Autodesk Inventor part; units mm, degrees
ref_plane "YZ Plane" through (0, 0, 0) normal (1, 0, 0) x (0, 1, 0)
ref_plane "XZ Plane" through (0, 0, 0) normal (0, 1, 0) x (-1, 0, 0)
ref_plane "XY Plane" through (0, 0, 0) normal (0, 0, 1) x (1, 0, 0)
sketch "Sketch1" plane through (0, 0, 0) normal (0, 1, 0) x (-1, 0, 0)
  circle A0 centre (0, 0) radius 95.25 construction
  circle A1 centre (0, 0) radius 120.65 construction
  line L0 (-69.6573, -120.65) -> (-139.3146, 0)
  line L1 (-139.3146, 0) -> (-69.6573, 120.65)
  line L2 (-69.6573, 120.65) -> (69.6573, 120.65)
  line L3 (69.6573, 120.65) -> (139.3146, 0)
  line L4 (139.3146, 0) -> (69.6573, -120.65)
  line L5 (69.6573, -120.65) -> (-69.6573, -120.65)
  line L6 (142.4896, 0) -> (71.2448, 123.3996)
  line L7 (71.2448, 123.3996) -> (-71.2448, 123.3996)
  line L8 (-71.2448, 123.3996) -> (-142.4896, 0)
  line L9 (-142.4896, 0) -> (-71.2448, -123.3996)
  line L10 (-71.2448, -123.3996) -> (71.2448, -123.3996)
  line L11 (71.2448, -123.3996) -> (142.4896, 0)
  dimension "d0" = 190.5
  dimension "d1" = 25.4
  dimension "d2" = 3.175
extrude "Extrusion1" add sketch "Sketch1" along normal blind 209.55 contours L0 L1 L2 L3 L4 L5 | L11 L10 L9 L8 L7 L6
shell "Shell1" thickness 3.175 removed faces 1 at (47.4965, 209.55, 0)
sketch "Sketch2" plane through (142.4896, 0, 0) normal (0.866, 0, 0.5) x (0.5, 0, -0.866)
  circle A0 centre (-71.2448, 50.8) radius 9.525
  line L0 (-142.4896, 0) -> (0, 0)
  point P0 (-71.2448, 0)
  point P1 (-71.2448, 0)
  dimension "d15" = 19.05
  dimension "d16" = 50.8
extrude "Extrusion2" cut sketch "Sketch2" against normal up to next
sketch "Sketch3" plane through (0, 0, 0) normal (0, -1, 0) x (1, 0, 0)
  line L0 (-71.2448, 123.3996) -> (71.2448, 123.3996)
  circle A0 centre (0, 103.232) radius 1.7526
  line L1 (142.4896, 0) -> (71.2448, -123.3996)
  line L2 (106.8672, -61.6998) -> (130.6924, -61.6998) construction
  line L3 (-71.2448, -123.3996) -> (-142.4896, 0)
  line L4 (-106.8672, -61.6998) -> (-83.042, -61.6998) construction
  circle A1 centre (-89.4016, -51.616) radius 1.7526
  circle A2 centre (89.4016, -51.616) radius 1.7526
  point P0 (0, 0)
  dimension "d20" = 3.5052
  dimension "d21" = 20.1676
  dimension "d26" = 3.5052
  dimension "d27" = 3.5052
  dimension "d28" = 20.1676
  dimension "d29" = 20.1676
extrude "Extrusion3" cut sketch "Sketch3" against normal blind 12.7
thread "Thread1"
thread "Thread2"
thread "Thread3"
sketch "Sketch4" plane through (71.2448, 0, -123.3996) normal (0, 0, -1) x (-1, 0, 0)
  line L0 (3.2998, 144.145) -> (139.1898, 144.145) construction
  line L1 (139.1898, 144.145) -> (139.1898, 8.255) construction
  line L2 (139.1898, 8.255) -> (3.2998, 8.255) construction
  line L3 (3.2998, 8.255) -> (3.2998, 144.145) construction
  line L4 (3.2998, 144.145) -> (139.1898, 8.255) construction
  line L5 (139.1898, 144.145) -> (3.2998, 8.255) construction
  line L6 (0, 0) -> (142.4896, 0)
  circle A0 centre (139.1898, 144.145) radius 1.7996
  circle A1 centre (3.2998, 144.145) radius 1.7996
  circle A2 centre (3.2998, 8.255) radius 1.7996
  circle A3 centre (139.1898, 8.255) radius 1.7996
  point P0 (71.2448, 0)
  point P1 (71.2448, 76.2)
  point P2 (71.2448, 76.2)
  point P3 (71.2448, 0)
  dimension "d38" = 135.89
  dimension "d39" = 76.2
  dimension "d40" = 3.5992
sketch "Sketch5" plane through (-142.4896, 0, 0) normal (-0.866, 0, -0.5) x (-0.5, 0, 0.866)
  line L0 (-139.1898, 144.145) -> (-3.2998, 144.145) construction
  line L1 (-3.2998, 144.145) -> (-3.2998, 8.255) construction
  line L2 (-3.2998, 8.255) -> (-139.1898, 8.255) construction
  line L3 (-139.1898, 8.255) -> (-139.1898, 144.145) construction
  line L4 (-139.1898, 144.145) -> (-3.2998, 8.255) construction
  line L5 (-3.2998, 144.145) -> (-139.1898, 8.255) construction
  line L6 (0, 0) -> (-142.4896, 0)
  circle A0 centre (-3.2998, 144.145) radius 1.7996
  circle A1 centre (-139.1898, 144.145) radius 1.7996
  circle A2 centre (-139.1898, 8.255) radius 1.7996
  circle A3 centre (-3.2998, 8.255) radius 1.7996
  line L7 (-142.4896, 0) -> (0, 0)
  point P0 (-71.2448, 0)
  point P1 (-71.2448, 0)
  point P2 (-71.2448, 76.2)
  point P3 (-71.2448, 76.2)
  point P4 (-71.2448, 0)
  point P5 (-71.2448, 0)
  point P6 (-71.2448, 76.2)
  point P7 (-71.2448, 0)
  dimension "d41" = 135.89
  dimension "d42" = 76.2
  dimension "d43" = 3.5992
extrude "Extrusion4" cut sketch "Sketch4" against normal up to next
extrude "Extrusion5" cut sketch "Sketch5" against normal up to next
equation "\"d5\" = d2"
properties part number "HS-01" material "Aluminum 6061 Painted"
Here's how the part is built. I have some questions about the finished solid (model axes, mm). A direction names the side the tool comes from. Coordinates: 2 decimals unless noted, no trailing zeros. Loops run counter-clockwise (first coordinate to the right, second up) from the corner with the lowest first, then second, coordinate; pieces in that order, holes last. Notation, with made-up numbers: (17.25, 72) - (21.25, 72) arc R21 cw to (21.25, 100) - close; hole circle Ø6 at (28.25, 6.5). An arc over 180 degrees is marked (long way). Return JSON: item names as keys, results as strings. Group by question number.
Item 1: If we section it at A-A on y = 94: Write out the boundary of the cut face in (x, z).
Item 2: On a 3-axis mill with a long thin cutter (end or side, diameter ignored), from which of +Z, -Z, +X, -X, +Y, -Y can I reach the whole of each face in a straight line? I mean faces 5 (the face through (103.632, 104.918, 60.954)), 6 (the face through (107.366, 103.308, -60.836)). Say none if no direction works.
Item 3: If we section it at B-B on z = -34: Write out the boundary of the cut face in (x, y) (3 decimals).
Item 4: Will these pins go through, and if not, where does the flat tip stop? P1, Ø4, axis at x = -81.5, y = 25, coming from the -Z side; P2, Ø2, axis at x = -94.5, z = 39.5, coming from the +Y side (3 decimals); P3, Ø1, axis at x = -77, y = 31, coming from the +Z side; P4, Ø2, axis at x = 0, z = 103.232, coming from the +Y side.
Item 5: If we section it at C-C on x = 79.5: Write out the boundary of the cut face in (y, z) (3 decimals).
Item 6: We'd pull the mould along Z, two halves only. Please class faces 1 (the face through (2, 0, 2)), 2 (the face through (1, 103, -123.4)), 3 (the face through (2, 3.175, 2)), 4 (the face through (-107.366, 103.308, 60.836)): +Z half, -Z half, draft (parallel to the pull), parting line (faces both ways), or undercut.
Item 7: I need wall thicknesses on line 1 (Z direction, x = -41, y = 178.5); line 2 (Y direction, x = 86, z = 65.5) (3 decimals); line 3 (X direction, y = 86.5, z = 17). Which ranges of each line are inside material? Lowest first, please. Write a range as from..to.
Calculated:
{
 "1": {"outline": "(-142.49, 0) - (-71.24, -123.4) - (71.24, -123.4) - (142.49, 0) - (71.24, 123.4) - (-71.24, 123.4) - close; hole (-138.82, 0) - (-69.41, -120.22) - (69.41, -120.22) - (138.82, 0) - (69.41, 120.22) - (-69.41, 120.22) - close"},
 "2": {"face 5": "+Y", "face 6": "-Z, +X, +Y, -Y"},
 "3": {"outline": "(-122.86, 0) - (122.86, 0) - (122.86, 209.55) - (119.194, 209.55) - (119.194, 3.175) - (-119.194, 3.175) - (-119.194, 209.55) - (-122.86, 209.55) - close"},
 "4": {"P1": "stops at z = -109.1", "P2": "stops at y = 3.175", "P3": "stops at z = 114.3", "P4": "passes through"},
 "5": {"outline": "(0, -109.101) - (209.55, -109.101) - (209.55, -102.751) - (3.175, -102.751) - (3.175, 102.751) - (209.55, 102.751) - (209.55, 109.101) - (0, 109.101) - close"},
 "6": {"face 1": "draft", "face 2": "-Z half", "face 3": "undercut", "face 4": "+Z half"},
 "7": {"line 1": "z = -123.4..-120.22, 120.22..123.4", "line 2": "y = 0..3.175", "line 3": "x = -132.67..-129.01, 129.01..132.67"}
}
